from build123d import *

# Parameters (mm, degrees)
SKETCH1_W           = 102
SKETCH1_H           = 80
SKETCH1_W_2         = 85
SKETCH1_H_2         = 65
BOSS_EXTRUDE1_DEPTH = 2
FILLET2_R           = 5
SKETCH2_R           = 1.6
CUT_EXTRUDE1_DEPTH  = 64.5


with BuildPart() as part:
    # Sketch1 → Boss-Extrude1 (new body)
    with BuildSketch(Plane(origin=(0, 0, 0), x_dir=(1, 0, 0), z_dir=(0, 1, 0))):
        Rectangle(SKETCH1_W, SKETCH1_H)
        Rectangle(SKETCH1_W_2, SKETCH1_H_2, mode=Mode.SUBTRACT)
    extrude(amount=BOSS_EXTRUDE1_DEPTH)

    # Fillet2
    fillet2_edges = [part.edges().sort_by_distance(p)[0] for p in [
        (-51, 1, 40),
        (-51, 1, -40),
        (51, 1, -40),
        (51, 1, 40),
    ]]
    fillet(fillet2_edges, radius=FILLET2_R)

    # Sketch2 → Cut-Extrude1 (cut, symmetric)
    with BuildSketch(Plane(origin=(0, 2, 0), x_dir=(1, 0, 0), z_dir=(0, 1, 0))):
        with Locations(Location((-47, -35, 0), (0, 0, 90))):
            Circle(SKETCH2_R)
        with Locations(Location((47, -35, 0), (0, 0, 90))):
            Circle(SKETCH2_R)
        with Locations(Location((47, 35, 0), (0, 0, 90))):
            Circle(SKETCH2_R)
        with Locations(Location((-47, 35, 0), (0, 0, 90))):
            Circle(SKETCH2_R)
    extrude(amount=CUT_EXTRUDE1_DEPTH, both=True, mode=Mode.SUBTRACT)


solid = part.part
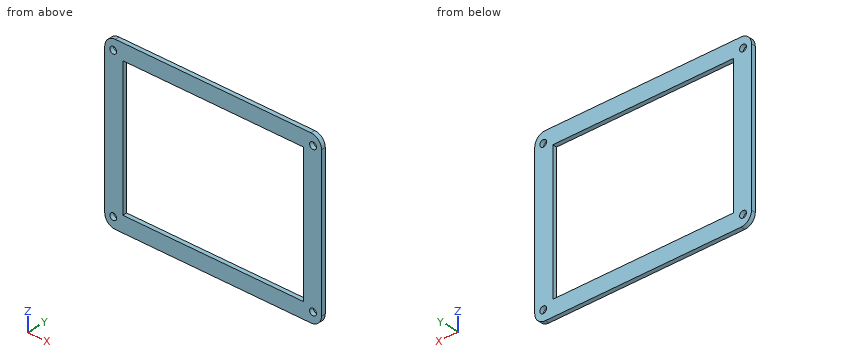
Geometry: final body of the model. Coordinates: model frame, mm. Coordinates: 2 decimals unless noted, no trailing zeros. Order: outer loops, then holes, each group sorted by start corner. A loop starts at its lowest first (then second) coordinate and runs counter-clockwise, first axis right, second up. Notation, with made-up numbers: M 10.25,30.5 L 20.25,30.5 A15 cw 20.25,50.5 Z; hole C -13,-29 d1. An arc over 180 degrees is marked long. One line per question, with ' | ' between items. Start each with the question number.
Item 1: Ray query, probe 1 along X at (y, z) = (0.7, -35); probe 2 along Z at (x, y) = (-25.5, 1.15); probe 3 along X at (y, z) = (1.75, -15). Return the intervals inside material, ascending. Write a range as [from, to].
Item 2: Cut plane A-A, the plane z = 10. Return the cut outline in (x, y).
Item 3: Cut plane C-C, the plane x = 38.5. Return the cut outline in (y, z), then the cut area to 3 significant figures.
Item 4: Cut plane B-B, the plane y = 0.95. Return the cut outline in (x, z), then the cut area to 3 significant figures.
A:
1) probe 1: x = [-51, -48.6], [-45.4, 45.4], [48.6, 51] | probe 2: z = [-40, -32.5], [32.5, 40] | probe 3: x = [-51, -42.5], [42.5, 51]
2) outline: M -51,0 L -42.5,0 L -42.5,2 L -51,2 Z; M 42.5,0 L 51,0 L 51,2 L 42.5,2 Z
3) outline: M 0,-40 L 2,-40 L 2,-32.5 L 0,-32.5 Z; M 0,32.5 L 2,32.5 L 2,40 L 0,40 Z | area: 30.0 mm2
4) outline: M -51,-35 A5 ccw -46,-40 L 46,-40 A5 ccw 51,-35 L 51,35 A5 ccw 46,40 L -46,40 A5 ccw -51,35 Z; hole C -47,-35 d3.2; hole C -47,35 d3.2; hole M -42.5,-32.5 L 42.5,-32.5 L 42.5,32.5 L -42.5,32.5 Z; hole C 47,-35 d3.2; hole C 47,35 d3.2 | area: 2,580 mm2
